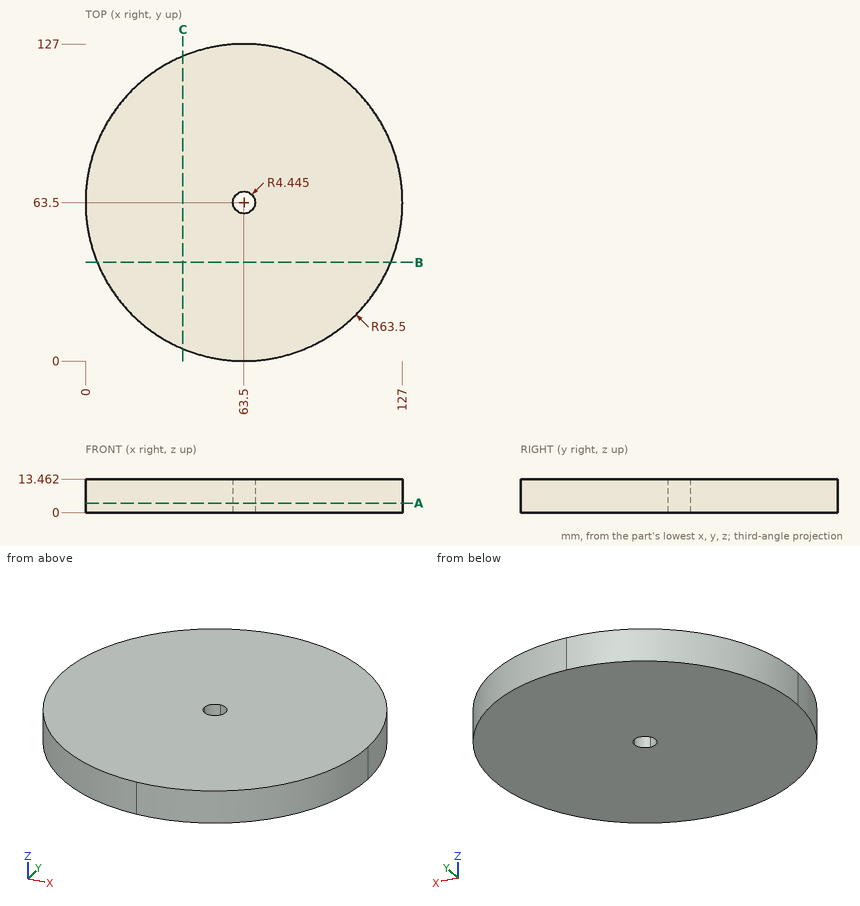
Could you check a few things on this drawing? It's one solid part, dimensions in mm from its lowest x, y, z. Give positions to 0.01 mm unless a question says otherwise; leave off trailing zeros. Write each loop counter-clockwise with the first axis right and the second up, starting at its lowest first coordinate (ties: lowest second). Pieces come first, ordered by that corner, then holes. Notation, with made-up numbers: (-9, -35) -> (28, -35) arc R16 ccw to (28, -11) -> close; hole circle Ø6 at (69.5, -5.5). An arc over 180 degrees is marked (long way). Write each question's results on one line, items separated by ' | '.
1. I want a section at B-B, the plane y = 39.5. Write out the boundary of the cut face in (x, z).
Check sheet entries:
outline: (4.71, 0) -> (122.29, 0) -> (122.29, 13.46) -> (4.71, 13.46) -> close
2. I want a section at A-A, the plane z = 3.75. Write out the boundary of the cut face in (x, y) (3 decimals), then the cut area to 3 significant figures.
Check sheet entries:
outline: (0, 63.5) arc R63.5 ccw to (63.5, 0) arc R63.5 ccw to (127, 63.5) arc R63.5 ccw to (63.5, 127) arc R63.5 ccw to start; hole (59.055, 63.5) arc R4.445 ccw to (63.5, 59.055) arc R4.445 ccw to (67.945, 63.5) arc R4.445 ccw to (63.5, 67.945) arc R4.445 ccw to start | area: 12,600 mm²
3. I need wall thicknesses on L1, parallel to X at y = 13.5, z = 3.5; L2, parallel to Y at x = 40, z = 5.25; L3, parallel to X at y = 91, z = 12. Which ranges of each line are inside material? Lowest first, please.
Check sheet entries:
L1: x = 24.36 to 102.64 | L2: y = 4.51 to 122.49 | L3: x = 6.26 to 120.74
4. Will these pins go through, and if not, where does the flat tip stop? pin 1 Ø5 at (y, z) = (70.5, 8.5) entering from +X; pin 2 Ø4 at (y, z) = (83, 7.5) entering from -X; pin 3 Ø8 at (x, z) = (99.5, 8.5) entering from +Y; pin 4 Ø6 at (x, y) = (51, 43) entering from -Z.
Check sheet entries:
pin 1: stops at x = 126.84 | pin 2: stops at x = 2.46 | pin 3: stops at y = 118.35 | pin 4: stops at z = 0
5. I want a section at C-C, the plane x = 39. Write out the boundary of the cut face in (y, z).
Check sheet entries:
outline: (4.92, 0) -> (122.08, 0) -> (122.08, 13.46) -> (4.92, 13.46) -> close
